```python
from build123d import *

# Parameters (mm, degrees)
BASE_EXTRUDE_DEPTH      = 44.45
CUT_EXTRUDE1_DEPTH      = 109.236398037
FILLET1_R               = 3.175
HOLE1_START             = 23.8125
HOLE1_OUTLINE_R         = 3.175
HOLE1_DEPTH             = 20.6375
LPATTERN1_COUNT         = 2
LPATTERN1_PITCH         = 76.2
MIRROR1_START           = 23.8125
MIRROR1_COPY_1_SKETCH_R = 3.175
MIRROR1_COPY_1_DEPTH    = 20.6375
MIRROR1_COPY_2_SKETCH_R = 3.175
MIRROR1_COPY_2_DEPTH    = 20.6375
HOLE2_START             = 26.9875
HOLE2_OUTLINE_R         = 3.9751
HOLE2_DEPTH             = 17.4625


# Read off the part's stored shape, not the designer's step: Hole1, Hole2
with BuildPart() as part:
    # Sketch1 → Base-Extrude (new, symmetric)
    with BuildSketch(Plane(origin=(0, 0, 0), x_dir=(0, 0, -1), z_dir=(1, 0, 0))):
        with BuildLine():
            Line((-44.45, 0), (44.45, 0))
            Line((44.45, 0), (44.45, -16.643244248))
            ThreePointArc((44.45, -16.643244248), (0, -42.8498), (-44.45, -16.643244248))
            Line((-44.45, -16.643244248), (-44.45, 0))
        make_face()
    extrude(amount=BASE_EXTRUDE_DEPTH, both=True)

    # Sketch2 → Cut-Extrude1 (cut, through all)
    with BuildSketch(Plane.XY.offset(44.45)):
        with BuildLine():
            Line((-173.766299507, 128.569272459), (-34.452576283, 0))
            ThreePointArc((-34.452576283, 0), (0, -13.468244248), (34.452576283, 0))
            Line((34.452576283, 0), (173.766299507, 128.569272459))
            Line((173.766299507, 128.569272459), (173.766299507, 507.717640776))
            Line((173.766299507, 507.717640776), (-173.766299507, 507.717640776))
            Line((-173.766299507, 507.717640776), (-173.766299507, 128.569272459))
        make_face()
    extrude(amount=-CUT_EXTRUDE1_DEPTH, mode=Mode.SUBTRACT)

    # Fillet1
    fillet1_edges = [part.edges().sort_by_distance(p)[0] for p in [
        (44.45, 0, 0),
        (-44.45, 0, 0),
    ]]
    fillet(fillet1_edges, radius=FILLET1_R)

    # Hole1 outline → Hole1 (cut)
    with BuildSketch(Plane.XY.offset(HOLE1_START)):
        with Locations((-38.1, -7.1374)):
            Circle(HOLE1_OUTLINE_R)
    hole1 = extrude(amount=HOLE1_DEPTH, mode=Mode.SUBTRACT)

    # LPattern1: Hole1 ×2
    with Locations(*[(i * LPATTERN1_PITCH, 0, 0) for i in range(1, LPATTERN1_COUNT)]):
        add(hole1, mode=Mode.SUBTRACT)

    # Mirror1 copy 1 sketch → Mirror1 copy 1 (cut)
    with BuildSketch(Plane(origin=(76.2, 0, 0), x_dir=(1, 0, 0), z_dir=(0, 0, -1)).offset(MIRROR1_START)):
        with Locations((-38.1, 7.1374)):
            Circle(MIRROR1_COPY_1_SKETCH_R)
    extrude(amount=MIRROR1_COPY_1_DEPTH, mode=Mode.SUBTRACT)

    # Mirror1 copy 2 sketch → Mirror1 copy 2 (cut)
    with BuildSketch(Plane(origin=(0, 0, 0), x_dir=(1, 0, 0), z_dir=(0, 0, -1)).offset(MIRROR1_START)):
        with Locations((-38.1, 7.1374)):
            Circle(MIRROR1_COPY_2_SKETCH_R)
    extrude(amount=MIRROR1_COPY_2_DEPTH, mode=Mode.SUBTRACT)

    # Hole2 outline → Hole2 (cut)
    with BuildSketch(Plane.YZ.offset(HOLE2_START)):
        with Locations((-35.179, 0)):
            Circle(HOLE2_OUTLINE_R)
    hole2 = extrude(amount=HOLE2_DEPTH, mode=Mode.SUBTRACT)

    # Mirror2: Hole2 across plane
    add(hole2.mirror(Plane(origin=(0, 0, 0), x_dir=(0, 0, 1), z_dir=(1, 0, 0))), mode=Mode.SUBTRACT)


solid = part.part
```
CAD build for the part. Positions are in the model's coordinates, mm. A direction names the side the tool comes from. Round coordinates to 2 decimals unless told otherwise and drop trailing zeros. Order: outer loops, then holes, each group sorted by start corner. A loop starts at its lowest first (then second) coordinate and runs counter-clockwise, first axis right, second up. Notation, with made-up numbers: (-14.5, -8) - (8.5, -8) arc R31 cw to (8.5, 21) - close; hole circle Ø1 at (-10, -13.5). An arc over 180 degrees is marked (long way). Answer as CSV lines item,"result". Start each with the question number.
1. Saw through at B-B, the plane y = -6. Write the cut outline in (x, z), and give its area (3 significant figures).
2. Saw through at D-D, the plane z = -25.5. Write the cut outline in (x, y) (3 decimals).
3. Pin check, flat tips, straight feed: pin 1 (6.5 mm diameter, centred on y = -35.179, z = 0, fed in from -X); pin 2 (6.5 mm diameter, centred on y = -35.5, z = 0, fed in from +X); pin 3 (5 mm diameter, centred on x = 38.1, y = -7.14, fed in from -Z). Stop position of each tip, or through.
4. Pull direction X, two halves, no side cores. Call faces 5 (the face through (-38, 0, 1)), 6 (the face through (-0.53, -13.465, 0.622)), 7 (the face through (-43.5, -0.91, -0.62)): +X half, -X half, draft (parallel to the pull), parting line (faces both ways), or undercut.
5. Drill centre lines: L1, parallel to X at y = -7.5, z = -23; L2, parallel to X at y = -9, z = -19; L3, parallel to Z at x = -30.5, y = -24.5. Where is each one in solid material? Low to high. Write a range as [from, to].
6. Saw through at A-A, the plane x = 38.1. Write the cut outline in (y, z), and give its area (3 significant figures).
7. Tool access for faces 1 (the face through (26.988, -35, 0)), 2 (the face through (-35.597, -31.507, -1.522)), 3 (the face through (34.928, -6.998, 33.987)), 4 (the face through (37.41, -4.04, -33.99)): list every direction of +Z, -Z, +X, -X, +Y, -Y with a clear straight run to the whole face (end or side of a thin tool).
Model answer:
1,outline,"(-44.45, -44.45) - (-41.06, -44.45) - (-41.06, -23.81) - (-35.14, -23.81) - (-35.14, -44.45) - (-26.51, -44.45) - (-26.51, 44.45) - (-35.14, 44.45) - (-35.14, 23.81) - (-41.06, 23.81) - (-41.06, 44.45) - (-44.45, 44.45) - close; (26.51, -44.45) - (35.14, -44.45) - (35.14, -23.81) - (41.06, -23.81) - (41.06, -44.45) - (44.45, -44.45) - (44.45, 44.45) - (41.06, 44.45) - (41.06, 23.81) - (35.14, 23.81) - (35.14, 44.45) - (26.51, 44.45) - close"
1,area,"2,700 mm²"
2,outline,"(-44.45, -35.986) - (44.45, -35.986) - (44.45, -3.175) arc R3.175 ccw to (41.275, 0) - (34.453, 0) arc R50.8 cw to (-34.453, 0) - (-41.275, 0) arc R3.175 ccw to (-44.45, -3.175) - close; hole circle Ø6.35 at (-38.1, -7.137); hole circle Ø6.35 at (38.1, -7.137)"
3,pin 1,"stops at x = -26.99"
3,pin 2,"stops at x = 26.99"
3,pin 3,"stops at z = -23.81"
4,face 5,"draft"
4,face 6,"undercut"
4,face 7,"-X half"
5,L1,"x = [-44.45, -23.89], [23.89, 44.45]"
5,L2,"x = [-44.45, -20.83], [20.83, 44.45]"
5,L3,"z = [-39.08, 39.08]"
6,outline,"(-16.64, -44.45) - (-10.31, -44.45) - (-10.31, -23.81) - (-3.96, -23.81) - (-3.96, -44.45) - (0, -44.45) - (0, 44.45) - (-3.96, 44.45) - (-3.96, 23.81) - (-10.31, 23.81) - (-10.31, 44.45) - (-16.64, 44.45) arc R50.8 ccw to start; hole circle Ø7.95 at (-35.18, 0)"
6,area,"2,820 mm²"
7,face 1,"+X"
7,face 2,"-X"
7,face 3,"+Z"
7,face 4,"-Z"
